CAD build for the part. Positions are in the model's coordinates, mm. A direction names the side the tool comes from. Give positions to 0.01 mm unless a question says otherwise; leave off trailing zeros. Write each loop counter-clockwise with the first axis right and the second up, starting at its lowest first coordinate (ties: lowest second). Pieces come first, ordered by that corner, then holes. Notation, with made-up numbers: (3.25, 53.25) -> (40.25, 53.25) arc R15 cw to (40.25, 65.25) -> close; hole circle Ø8 at (-4.5, 56). An arc over 180 degrees is marked (long way). Answer as a JSON object with one key per item and string values.
```python
from build123d import *

# Parameters (mm, degrees)
F1_DEPTH = 4.5
F2_R     = 11
F2_R_2   = 24
F3_DEPTH = 50
F2_R_3   = 2.5
F4_DEPTH = 25
F5_DEPTH = 3.5
F6_DEPTH = 2
F7_R     = 25.25
F8_DEPTH = 4


# Not quite as in the source:
# - a feature names something its author has since deleted; it is built from what else it names


with BuildPart() as f1:
    # F0 (on Top) → F1 (new body)
    with BuildSketch(Plane.XY):
        Polygon((-46.0190125704, -8.1893682778), (-110.0190125704, -8.1893682778), (-117.0190125704, -41.6893682778), (-110.0190125704, -77.6893682778), (-46.0190125704, -77.6893682778), (-39.0190125704, -41.6893682778), align=None)
    extrude(amount=F1_DEPTH)

    # F2 (on face) → F3 (cut)
    with BuildSketch(Plane.XY.offset(4.5)):
        with Locations((36.7125935962, -5.1025906342)):
            Circle(F2_R)
        with Locations((63.6127434798, -2.782690585)):
            Circle(F2_R)
        with Locations((-78.0190125704, -51.4393682778)):
            Circle(F2_R_2)
    extrude(amount=-F3_DEPTH, mode=Mode.SUBTRACT)

    # F2 (on face) → F4 (cut)
    with BuildSketch(Plane.XY.offset(4.5)):
        with Locations((-103.5190125704, -14.1893682778)):
            Circle(F2_R_3)
        with Locations((-52.0190125704, -15.1893682778)):
            Circle(F2_R_3)
        with Locations((-105.5190125704, -70.6893682778)):
            Circle(F2_R_3)
        with Locations((-50.5190125704, -70.6893682778)):
            Circle(F2_R_3)
    extrude(amount=-F4_DEPTH, mode=Mode.SUBTRACT)

    # F2 (on face) → F5 (cut)
    with BuildSketch(Plane.XY.offset(4.5)):
        with BuildLine():
            Line((-110.0190125704, -8.1893682778), (-111.7083286904, -16.2739525667))
            ThreePointArc((-111.7083286904, -16.2739525667), (-103.2870621366, -20.4161997132), (-97.4153326836, -13.0950840178))
            ThreePointArc((-97.4153326836, -13.0950840178), (-97.8868841728, -10.4776594188), (-99.2422424253, -8.1893682778))
            Line((-99.2422424253, -8.1893682778), (-110.0190125704, -8.1893682778))
        make_face()
        with Locations((-103.5190125704, -14.1893682778)):
            Circle(F2_R_3, mode=Mode.SUBTRACT)
        with BuildLine():
            Line((-46.0190125704, -8.1893682778), (-55.7181574473, -8.1893682778))
            ThreePointArc((-55.7181574473, -8.1893682778), (-55.3158791173, -19.6211139555), (-44.1027782894, -17.3599180513))
            Line((-44.1027782894, -17.3599180513), (-46.0190125704, -8.1893682778))
        make_face()
        with Locations((-52.0190125704, -15.1893682778)):
            Circle(F2_R_3, mode=Mode.SUBTRACT)
        with BuildLine():
            ThreePointArc((-101.3837870838, -77.6893682778), (-99.5825379735, -75.1790324483), (-98.9461190179, -72.1555815644))
            ThreePointArc((-98.9461190179, -72.1555815644), (-103.7878144934, -65.1424925834), (-112.0616968993, -67.1841345861))
            Line((-112.0616968993, -67.1841345861), (-110.0190125704, -77.6893682778))
            Line((-110.0190125704, -77.6893682778), (-101.3837870838, -77.6893682778))
        make_face()
        with Locations((-105.5190125704, -70.6893682778)):
            Circle(F2_R_3, mode=Mode.SUBTRACT)
        with BuildLine():
            ThreePointArc((-43.9012732129, -66.7981372962), (-54.8452929266, -66.7661737817), (-54.1697108353, -77.6893682778))
            Line((-54.1697108353, -77.6893682778), (-46.0190125704, -77.6893682778))
            Line((-46.0190125704, -77.6893682778), (-43.9012732129, -66.7981372962))
        make_face()
        with Locations((-50.5190125704, -70.6893682778)):
            Circle(F2_R_3, mode=Mode.SUBTRACT)
    extrude(amount=-F5_DEPTH, mode=Mode.SUBTRACT)

    # F2 (on face) → F6 (cut)
    with BuildSketch(Plane.XY.offset(4.5)):
        with Locations((-78.0190125704, -51.4393682778)):
            Circle(F2_R_2)
    extrude(amount=-F6_DEPTH, mode=Mode.SUBTRACT)

    # F7 (on face) → F8 (cut)
    with BuildSketch(Plane(origin=(0, 0, 0), x_dir=(1, 0, 0), z_dir=(0, 0, -1))):
        with Locations((-78.0190125704, 51.4393682778)):
            Circle(F7_R)
    extrude(amount=-F8_DEPTH, mode=Mode.SUBTRACT)


solid = f1.part
```
1) Slice it at A-A (y = -47). List the corners of the cut face in (x, z), then the cut area to 3 significant figures.
Model answer:
{"outline": "(-115.99, 0) -> (-102.88, 0) -> (-102.88, 4) -> (-101.6, 4) -> (-101.6, 4.5) -> (-115.99, 4.5) -> close; (-54.43, 4) -> (-53.16, 4) -> (-53.16, 0) -> (-40.05, 0) -> (-40.05, 4.5) -> (-54.43, 4.5) -> close", "area": "119 mm2"}
2) Pin check, flat tips, straight feed: pin 1 (12 mm diameter, centred on x = -50.67, y = -13.73, fed in from +Z); pin 2 (1.5 mm diameter, centred on y = -62.5, z = 2.5, fed in from -X); pin 3 (2 mm diameter, centred on y = -35, z = 4, fed in from +X). Stop position of each tip, or through.
Model answer:
{"pin 1": "stops at z = 1", "pin 2": "stops at x = -113.12", "pin 3": "stops at x = -40.21"}
3) Slice it at C-C (z = 2.8). List the corners of the cut face in (x, y), then the cut area to 3 significant figures.
Model answer:
{"outline": "(-117.02, -41.69) -> (-112.06, -67.18) arc R7.5 cw (long way) to (-101.38, -77.69) -> (-54.17, -77.69) arc R7.5 cw (long way) to (-43.9, -66.8) -> (-39.02, -41.69) -> (-44.1, -17.36) arc R7.5 cw (long way) to (-55.72, -8.19) -> (-99.24, -8.19) arc R7.5 cw (long way) to (-111.71, -16.27) -> close; hole circle Ø50.5 at (-78.02, -51.44)", "area": "2,350 mm2"}
4) Wall check: probe 1 along Y at (x, z) = (-55, 2.85); probe 2 along X at (y, z) = (-70, 0.3); probe 3 along Z at (x, y) = (-99.5, -14). Give the ranges that are in metal, low to high.
Model answer:
{"probe 1": "y = -77.69 to -76.89, -66.94 to -61.82, -41.06 to -19.86", "probe 2": "x = -111.51 to -107.92, -103.12 to -95.14, -60.9 to -52.92, -48.12 to -44.52", "probe 3": "z = 0 to 1"}
5) Mould opens along Y. For faces 1 (the flat face through (-79, -27, 4.5)), 2 (the flat face through (-114.346, -55.437, 2.218)), 3 (the cylindrical face through (-107.503, -72.211, 0.507)) say: released by +Y, released by -Y, zero draft, split by the parting line, or undercut.
Model answer:
{"face 1": "zero draft", "face 2": "released by -Y", "face 3": "undercut"}
6) Slice it at B-B (x = -86). List the corners of the cut face in (y, z), then the cut area to 3 significant figures.
Model answer:
{"outline": "(-77.69, 0) -> (-75.39, 0) -> (-75.39, 4) -> (-74.07, 4) -> (-74.07, 4.5) -> (-77.69, 4.5) -> close; (-28.81, 4) -> (-27.48, 4) -> (-27.48, 0) -> (-8.19, 0) -> (-8.19, 4.5) -> (-28.81, 4.5) -> close", "area": "98.5 mm2"}
7) 3-axis set-ups, long thin cutter, end or side, ignore diameter. For faces 4 (the flat face through (-114.25, -28.43, 2.22)), 5 (the cylindrical face through (-54.726, -66.643, 2.774)), 6 (the cylindrical face through (-53.935, -59.024, 1.972)): which of +Z, -Z, +X, -X, +Y, -Y reach the whole face in a straight line?
Model answer:
{"face 4": "+Z, -Z, -X, +Y", "face 5": "+Z", "face 6": "-Z"}
